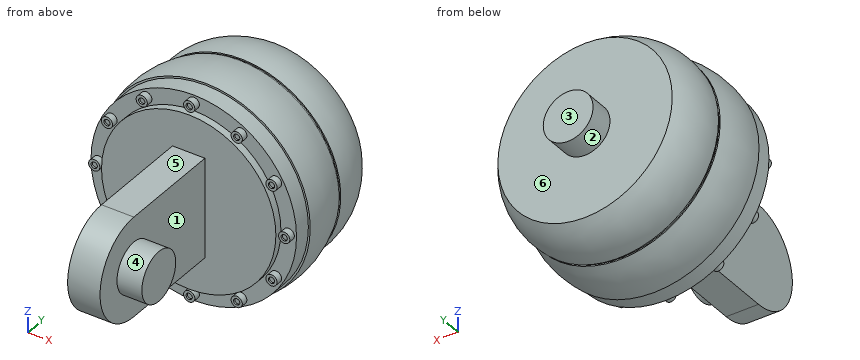
```python
from build123d import *

# Parameters (mm, degrees)
SKETCH2_R           = 39.5
BOSS_EXTRUDE1_DEPTH = 1
SKETCH5_R           = 41.25
BOSS_EXTRUDE2_DEPTH = 7
SKETCH6_R           = 35
BOSS_EXTRUDE3_DEPTH = 3
BOSS_EXTRUDE4_DEPTH = 2.7
SKETCH8_R           = 1.25
CUT_EXTRUDE1_DEPTH  = 0.7
CIRPATTERN1_COUNT   = 12
SKETCH9_W           = 13
SKETCH9_H           = 40
BOSS_EXTRUDE5_DEPTH = 42
BOSS_EXTRUDE7_DEPTH = 13
SKETCH13_R          = 10
BOSS_EXTRUDE8_DEPTH = 10
SKETCH14_R          = 10
BOSS_EXTRUDE9_DEPTH = 10


with BuildPart() as part:
    # Sketch1 → Revolve1 (revolve)
    with BuildSketch(Plane.XY):
        with BuildLine():
            Line((0, 0), (-35, 0))
            ThreePointArc((-35, 0), (-39.657515479, -9.46062113), (-40, -20))
            Line((-40, -20), (0, -20))
            Line((0, -20), (0, 0))
        make_face()
    revolve(axis=Axis((0, 0, 0), (0, -1, 0)))

    # Sketch2 → Boss-Extrude1 (add)
    with BuildSketch(Plane.XZ.offset(20)):
        Circle(SKETCH2_R)
    extrude(amount=BOSS_EXTRUDE1_DEPTH)

    # Sketch4 → Revolve2 (revolve)
    with BuildSketch(Plane.XY):
        with BuildLine():
            Line((0, -21), (0, -41))
            Line((0, -41), (-42, -41))
            ThreePointArc((-42, -41), (-42.384109041, -30.861589096), (-40, -21))
            Line((-40, -21), (0, -21))
        make_face()
    revolve(axis=Axis((0, -21, 0), (0, -1, 0)))

    # Sketch5 → Boss-Extrude2 (add)
    with BuildSketch(Plane.XZ.offset(41)):
        Circle(SKETCH5_R)
    extrude(amount=BOSS_EXTRUDE2_DEPTH)

    # Sketch6 → Boss-Extrude3 (add)
    with BuildSketch(Plane.XZ.offset(48)):
        Circle(SKETCH6_R)
    extrude(amount=BOSS_EXTRUDE3_DEPTH)

    # Sketch7 → Boss-Extrude4 (add)
    with BuildSketch(Plane(origin=(0, -48, 0), x_dir=(-1, 0, 0), z_dir=(0, -1, 0))):
        with BuildLine():
            ThreePointArc((-40.375, 0), (-38.125, -2.25), (-35.875, 0))
            Line((-35.875, 0), (-40.375, 0))
        make_face()
        with BuildLine():
            Line((-40.375, 0), (-35.875, 0))
            ThreePointArc((-35.875, 0), (-38.125, 2.25), (-40.375, 0))
        make_face()
    boss_extrude4 = extrude(amount=BOSS_EXTRUDE4_DEPTH)

    # Sketch8 → Cut-Extrude1 (cut)
    with BuildSketch(Plane.XZ.offset(50.7)):
        with Locations((38.125, 0)):
            Circle(SKETCH8_R)
    cut_extrude1 = extrude(amount=-CUT_EXTRUDE1_DEPTH, mode=Mode.SUBTRACT)

    # CirPattern1: Boss-Extrude4, Cut-Extrude1 ×12 about axis
    cirpattern1_axis = Axis((0, 0, 0), (0, 1, 0))
    for i in range(1, CIRPATTERN1_COUNT):
        add(boss_extrude4.rotate(cirpattern1_axis, i * 360 / CIRPATTERN1_COUNT))
        add(cut_extrude1.rotate(cirpattern1_axis, i * 360 / CIRPATTERN1_COUNT), mode=Mode.SUBTRACT)

    # Sketch9 → Boss-Extrude5 (add)
    with BuildSketch(Plane.XZ.offset(51)):
        Rectangle(SKETCH9_W, SKETCH9_H)
    extrude(amount=BOSS_EXTRUDE5_DEPTH)

    # Sketch12 → Boss-Extrude7 (add)
    with BuildSketch(Plane(origin=(6.5, 0, 0), x_dir=(0, 0, -1), z_dir=(1, 0, 0))):
        with BuildLine():
            Line((20, -93), (-20, -93))
            ThreePointArc((-20, -93), (0, -113), (20, -93))
        make_face()
    extrude(amount=-BOSS_EXTRUDE7_DEPTH)

    # Sketch13 → Boss-Extrude8 (add)
    with BuildSketch(Plane(origin=(6.5, 0, 0), x_dir=(0, 0, -1), z_dir=(1, 0, 0))):
        with Locations((0, -93)):
            Circle(SKETCH13_R)
    extrude(amount=BOSS_EXTRUDE8_DEPTH)

    # Sketch14 → Boss-Extrude9 (add)
    with BuildSketch(Plane(origin=(0, 0, 0), x_dir=(1, 0, 0), z_dir=(0, 1, 0))):
        Circle(SKETCH14_R)
    extrude(amount=BOSS_EXTRUDE9_DEPTH)


solid = part.part
```
CAD build for the part. Positions are in the model's coordinates, mm. Face numbers are marked on the shaded views. A direction names the side the tool comes from. Coordinates: 2 decimals unless noted, no trailing zeros. Order: outer loops, then holes, each group sorted by start corner. A loop starts at its lowest first (then second) coordinate and runs counter-clockwise, first axis right, second up. Notation, with made-up numbers: (7, 3) - (18, 3) arc R24 ccw to (18, 32) - close; hole circle Ø9 at (-4.75, 14). An arc over 180 degrees is marked (long way). Answer in a Markdown table with one row per item.
1. Slice it at A-A, the plane y = -97. List the corners of the cut face in (x, z), then the cut area to 3 significant figures.
Answer:
| item | result |
|---|---|
| outline | (-6.5, -19.6) - (6.5, -19.6) - (6.5, -9.17) - (16.5, -9.17) - (16.5, 9.17) - (6.5, 9.17) - (6.5, 19.6) - (-6.5, 19.6) - close |
| area | 693 mm² |
2. 3-axis set-ups, long thin cutter, end or side, ignore diameter. For the marked faces 4, 5 and 6: which of +Z, -Z, +X, -X, +Y, -Y reach the whole face in a straight line?
Answer:
| item | result |
|---|---|
| face 4 | +X |
| face 5 | +Z, +X, -X, -Y |
| face 6 | +Y |
3. Drill centre lines: L1, parallel to X at y = -72.5, z = 5.5; L2, parallel to Y at x = -25.5, z = -1; L3, parallel to Z at x = -8.5, y = -44.5. Where is each one in solid material? Low to high. Write a range as from..to.
Answer:
| item | result |
|---|---|
| L1 | -6.5..6.5 |
| L2 | -51..0 |
| L3 | -40.36..40.36 |
4. Flat gauge pins, fed straight in: P1, Ø5, axis at x = -19, z = -32, coming from the -Y side; P2, Ø10, axis at x = 24, z = -13, coming from the +Y side; P3, Ø2, axis at x = -19.06, z = -33.02, coming from the -Y side. Where does each tip first touch, or does it go through?
Answer:
| item | result |
|---|---|
| P1 | y = -51 |
| P2 | y = 0 |
| P3 | y = -50 |
5. Pull direction X, two halves, no side cores. Call the marked faces 1, 2 and 3: +X half, -X half, draft (parallel to the pull), parting line (faces both ways), or undercut.
Answer:
| item | result |
|---|---|
| face 1 | +X half |
| face 2 | parting line |
| face 3 | draft |
